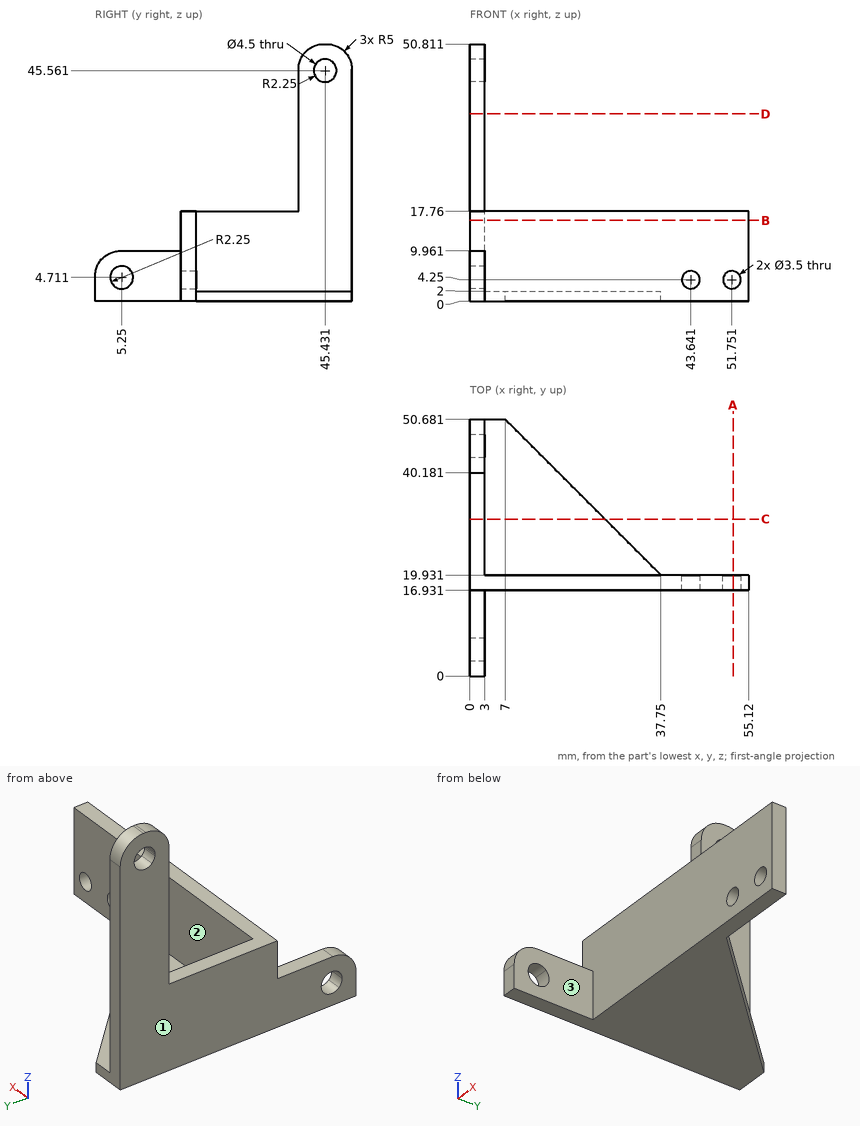
Here's the drawing with two shaded views (mm, measured from the low corner). I have some questions. A direction names the side the tool comes from. Give positions to 0.01 mm unless a question says otherwise; leave off trailing zeros. Loops run counter-clockwise (first coordinate to the right, second up) from the corner with the lowest first, then second, coordinate; pieces in that order, holes last. Notation, with made-up numbers: (83.25, 58) - (94.25, 58) arc R15 ccw to (94.25, 75) - close; hole circle Ø11 at (-17, -4.75). An arc over 180 degrees is marked (long way). Answer in a Markdown table with one row per item. Add a question column.
Q1. If we section it at C-C (y = 31): List the corners of the cut face in (x, z) for me, plus the area to 3 significant figures.
Q2. If we section it at D-D (z = 37): List the corners of the cut face in (x, y) for me, plus the area to 3 significant figures.
Q3. Please list where these lines run through material, in increasing order: L1, parallel to X at y = 17, z = 4; L2, parallel to X at y = 47, z = 22.5; L3, parallel to Y at x = 45, z = 13. Write a range as from..to.
Q4. If we section it at A-A (x = 52): List the corners of the cut face in (y, z) for me, plus the area to 3 significant figures.
Q5. For pin 1 (24.5 mm diameter, centred on y = 39.5, z = 29.5, fed in from +X); pin 2 (4 mm diameter, centred on x = 51.75, z = 4.25, fed in from +Y); pin 3 (3.5 mm diameter, centred on x = 1.5, y = 12.5, fed in from +Z); pin 4 (6 mm diameter, centred on x = 8, y = 8.5, fed in from +Z), each with a flat end and sliding along its axis, tell me the tip position at first contact or that it passes through.
Q6. If we section it at B-B (z = 16): List the corners of the cut face in (x, y) for me.
Q7. Which directions (+Z, -Z, +X, -X, +Y, -Y) give clear straight access to the entire face, cutting with the end or side of a thin tool? Please do the marked faces 1, 2 and 3.
The answers:
| question | item | result |
|---|---|---|
| 1 | outline | (0, 0) - (26.68, 0) - (26.68, 2) - (3, 2) - (3, 17.76) - (0, 17.76) - close |
| 1 | area | 101 mm^2 |
| 2 | outline | (0, 40.18) - (3, 40.18) - (3, 50.68) - (0, 50.68) - close |
| 2 | area | 31.5 mm^2 |
| 3 | L1 | x = 0..41.91, 45.37..50.02, 53.48..55.12 |
| 3 | L2 | x = 0..3 |
| 3 | L3 | y = 16.93..19.93 |
| 4 | outline | (16.93, 0) - (19.93, 0) - (19.93, 2.52) - (16.93, 2.52) - close; (16.93, 5.98) - (19.93, 5.98) - (19.93, 17.76) - (16.93, 17.76) - close |
| 4 | area | 42.9 mm^2 |
| 5 | pin 1 | stops at x = 3 |
| 5 | pin 2 | stops at y = 19.93 |
| 5 | pin 3 | stops at z = 9.96 |
| 5 | pin 4 | passes through |
| 6 | outline | (0, 16.93) - (55.12, 16.93) - (55.12, 19.93) - (3, 19.93) - (3, 50.68) - (0, 50.68) - close |
| 7 | face 1 | +Z, -Z, -X, +Y, -Y |
| 7 | face 2 | +Z, +X, +Y |
| 7 | face 3 | +Z, -Z, +X, -Y |
